Work out the finished part from the listing and answer in its coordinate system (mm). Give positions to 0.01 mm unless a question says otherwise; leave off trailing zeros. Order: outer loops, then holes, each group sorted by start corner. A loop starts at its lowest first (then second) coordinate and runs counter-clockwise, first axis right, second up. Notation, with made-up numbers: M 58.25,1.5 L 107.25,1.5 A12 cw 107.25,6.5 Z; hole C -5,15.25 d2. An arc over 180 degrees is marked long. One line per item, written item: value.
from build123d import *

# Parameters (mm, degrees)
SKETCH1_R               = 4.75
BOSS_EXTRUDE1_DEPTH     = 22
SKETCH2_R               = 6
BOSS_EXTRUDE2_DEPTH     = 1.5
CHAMFER1_SIZE           = 1
FILLET1_R               = 0.5
CUT_EXTRUDE1_DEPTH      = 25.984995545
CUT_EXTRUDE1_DEPTH_BACK = 25.984995545
SKETCH3_R               = 2


with BuildPart() as part:
    # Sketch1 → Boss-Extrude1 (new body)
    with BuildSketch(Plane(origin=(0, 0, 0), x_dir=(1, 0, 0), z_dir=(0, 1, 0))):
        with Locations(Location((0, 0, 0), (0, 0, 270))):
            Circle(SKETCH1_R)
    extrude(amount=BOSS_EXTRUDE1_DEPTH)

    # Sketch2 → Boss-Extrude2 (add)
    with BuildSketch(Plane(origin=(0, 22, 0), x_dir=(1, 0, 0), z_dir=(0, 1, 0))):
        with Locations(Location((0, 0, 0), (0, 0, 270))):
            Circle(SKETCH2_R)
    extrude(amount=BOSS_EXTRUDE2_DEPTH)

    # Chamfer1
    chamfer1_edges = [part.edges().sort_by_distance(p)[0] for p in [
        (0, 23.5, -6),
    ]]
    chamfer(chamfer1_edges, length=CHAMFER1_SIZE)

    # Fillet1
    fillet1_edges = [part.edges().sort_by_distance(p)[0] for p in [
        (0, 23.5, -5),
        (0, 22.5, -6),
    ]]
    fillet(fillet1_edges, radius=FILLET1_R)

    # Sketch3 → Cut-Extrude1 (cut, two sides: drawn at the far end of the back side and taken through both)
    with BuildSketch(Plane.XY.offset(-CUT_EXTRUDE1_DEPTH_BACK)):
        with Locations(Location((0, 6.5, 0), (0, 0, 90))):
            Circle(SKETCH3_R)
    extrude(amount=CUT_EXTRUDE1_DEPTH + CUT_EXTRUDE1_DEPTH_BACK, mode=Mode.SUBTRACT)


solid = part.part
(1) Section B-B, the plane y = 6.5 is taken. Give the vertices of the cut face in (x, z), then the cut area to 3 significant figures.
Findings:
outline: M -2,-4.31 L -2,4.31 A4.75 ccw Z; M 2,-4.31 A4.75 ccw 2,4.31 Z
area: 34.0 mm^2
(2) Find the intervals of material crossed by probe 1 along Y at (x, z) = (0, 1); probe 2 along X at (y, z) = (6.5, -0.5); probe 3 along Y at (x, z) = (1.75, 3.25), in increasing order. Write a range as from..to.
Findings:
probe 1: y = 0..4.5, 8.5..23.5
probe 2: x = -4.72..-2, 2..4.72
probe 3: y = 0..5.53, 7.47..23.5
(3) Section A-A, the plane y = 21.5 is taken. Give the vertices of the cut face in (x, z), then the cut area to 3 significant figures.
Findings:
outline: C 0,0 d9.5
area: 70.9 mm^2
(4) Given P1, Ø6, axis at y = 17.5, z = -1.5, coming from the -X side; P2, Ø2.5, axis at x = 0, y = 6.5, coming from the -Z side; P3, Ø3, axis at x = 0.5, z = -4.5, coming from the -Y side; P4, Ø3, axis at x = -2.5, y = 8, coming from the -Z side, each flat-ended and moving along its own axis, determine where each tip first touches the part or whether it passes through.
Findings:
P1: stops at x = -4.75
P2: passes through
P3: stops at y = 0
P4: stops at z = -4.64
(5) Determine the mould class of faces 1 (the flat face through (0, 0, 0)), 2 (the flat face through (0, 23.5, 0)), 3 (the cylindrical face through (1.2, 4.9, -0.1)) for opening direction Y: pulls with the +Y half, pulls with the -Y half, needs draft (parallel to the pull), parting line crosses it, or undercut.
Findings:
face 1: pulls with the -Y half
face 2: pulls with the +Y half
face 3: undercut
